Model file for the job. Use its own axes, mm. Face numbers are marked on the shaded views. A direction names the side the tool comes from. Give positions to 0.01 mm unless a question says otherwise; leave off trailing zeros. Write each loop counter-clockwise with the first axis right and the second up, starting at its lowest first coordinate (ties: lowest second). Pieces come first, ordered by that corner, then holes. Notation, with made-up numbers: (32.5, 5) - (38.5, 5) arc R29 cw to (38.5, 41) - close; hole circle Ø1 at (40.25, 60). An arc over 180 degrees is marked (long way). Use CSV: the item, a comma, the result in double quotes.
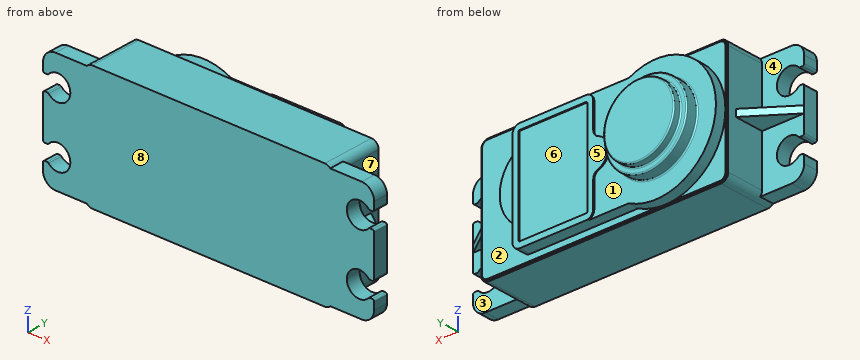
from build123d import *

# Parameters (mm, degrees)
CROQUIS1_W              = 41.6
CROQUIS1_H              = 20.6
SALIENTE_EXTRUIR1_DEPTH = 8.9
REDONDEO1_R             = 1.2
CROQUIS2_W              = 55.8
CROQUIS2_H              = 19.8
SALIENTE_EXTRUIR2_DEPTH = 2.45
REDONDEO2_R             = 2.1
CORTAR_EXTRUIR1_DEPTH   = 2.45
REDONDEO3_R             = 0.3
SALIENTE_EXTRUIR3_DEPTH = 0.2
CHAFL_N1_SIZE           = 0.1
SALIENTE_EXTRUIR4_DEPTH = 1.8
REDONDEO5_R             = 1.2
SALIENTE_EXTRUIR5_DEPTH = 0.2
CROQUIS11_R             = 6.95
SALIENTE_EXTRUIR6_DEPTH = 2
REDONDEO6_R             = 0.2
CROQUIS12_R             = 5.95
SALIENTE_EXTRUIR7_DEPTH = 1.3
REDONDEO7_R             = 0.2
SALIENTE_EXTRUIR8_DEPTH = 0.58


with BuildPart() as part:
    # Croquis1 → Saliente-Extruir1 (new body)
    with BuildSketch(Plane(origin=(0, 0, 0), x_dir=(1, 0, 0), z_dir=(0, 1, 0))):
        Rectangle(CROQUIS1_W, CROQUIS1_H)
    extrude(amount=SALIENTE_EXTRUIR1_DEPTH)

    # Redondeo1
    redondeo1_edges = [part.edges().sort_by_distance(p)[0] for p in [
        (20.8, 4.45, 10.3),
        (-20.8, 4.45, 10.3),
        (-20.8, 4.45, -10.3),
        (20.8, 4.45, -10.3),
    ]]
    fillet(redondeo1_edges, radius=REDONDEO1_R)

    # Croquis2 → Saliente-Extruir2 (add)
    with BuildSketch(Plane.XZ):
        Rectangle(CROQUIS2_W, CROQUIS2_H)
    extrude(amount=-SALIENTE_EXTRUIR2_DEPTH)

    # Redondeo2
    redondeo2_edges = [part.edges().sort_by_distance(p)[0] for p in [
        (-27.9, 1.225, -9.9),
        (-27.9, 1.225, 9.9),
        (27.9, 1.225, 9.9),
        (27.9, 1.225, -9.9),
    ]]
    fillet(redondeo2_edges, radius=REDONDEO2_R)

    # Croquis3 → Cortar-Extruir1 (cut)
    with BuildSketch(Plane.XZ):
        with BuildLine():
            Line((27.04924225, 6.3), (27.9, 6.3))
            Line((27.9, 6.3), (27.9, 3.7))
            Line((27.9, 3.7), (27.04924225, 3.7))
            ThreePointArc((27.04924225, 3.7), (23.3, 5), (27.04924225, 6.3))
        make_face()
        with BuildLine():
            Line((27.9, -6.3), (27.9, -3.7))
            Line((27.9, -3.7), (27.04924225, -3.7))
            ThreePointArc((27.04924225, -3.7), (23.3, -5), (27.04924225, -6.3))
            Line((27.04924225, -6.3), (27.9, -6.3))
        make_face()
        with BuildLine():
            Line((-27.04924225, -6.3), (-27.9, -6.3))
            Line((-27.9, -6.3), (-27.9, -3.7))
            Line((-27.9, -3.7), (-27.04924225, -3.7))
            ThreePointArc((-27.04924225, -3.7), (-23.3, -5), (-27.04924225, -6.3))
        make_face()
        with BuildLine():
            Line((-27.9, 6.3), (-27.9, 3.7))
            Line((-27.9, 3.7), (-27.04924225, 3.7))
            ThreePointArc((-27.04924225, 3.7), (-23.3, 5), (-27.04924225, 6.3))
            Line((-27.04924225, 6.3), (-27.9, 6.3))
        make_face()
    extrude(amount=-CORTAR_EXTRUIR1_DEPTH, mode=Mode.SUBTRACT)

    # Redondeo3
    redondeo3_edges = [part.edges().sort_by_distance(p)[0] for p in [
        (27.04924225, 1.225, 3.7),
        (27.04924225, 1.225, 6.3),
        (27.9, 1.225, 6.3),
        (27.9, 1.225, 3.7),
        (27.9, 1.225, -6.3),
        (27.04924225, 1.225, -6.3),
        (27.04924225, 1.225, -3.7),
        (27.9, 1.225, -3.7),
        (-27.9, 1.225, 6.3),
        (-27.04924225, 1.225, 6.3),
        (-27.04924225, 1.225, 3.7),
        (-27.9, 1.225, 3.7),
        (-27.9, 1.225, -6.3),
        (-27.9, 1.225, -3.7),
        (-27.04924225, 1.225, -3.7),
        (-27.04924225, 1.225, -6.3),
    ]]
    fillet(redondeo3_edges, radius=REDONDEO3_R)

    # Croquis4 → Saliente-Extruir3 (add)
    with BuildSketch(Plane(origin=(0, 8.9, 0), x_dir=(1, 0, 0), z_dir=(0, 1, 0))):
        with BuildLine():
            Line((20.6, -9.1), (20.6, 9.1))
            ThreePointArc((20.6, 9.1), (20.307106781, 9.807106781), (19.6, 10.1))
            Line((19.6, 10.1), (-19.6, 10.1))
            ThreePointArc((-19.6, 10.1), (-20.307106781, 9.807106781), (-20.6, 9.1))
            Line((-20.6, 9.1), (-20.6, -9.1))
            ThreePointArc((-20.6, -9.1), (-20.307106781, -9.807106781), (-19.6, -10.1))
            Line((-19.6, -10.1), (19.6, -10.1))
            ThreePointArc((19.6, -10.1), (20.307106781, -9.807106781), (20.6, -9.1))
        make_face()
    extrude(amount=SALIENTE_EXTRUIR3_DEPTH)

    # Chaflán1
    chafl_n1_edges = [part.edges().sort_by_distance(p)[0] for p in [
        (20.307106781, 9.1, -9.807106781),
        (0, 9.1, -10.1),
        (-20.307106781, 9.1, -9.807106781),
        (-20.6, 9.1, 0),
        (-20.307106781, 9.1, 9.807106781),
        (0, 9.1, 10.1),
        (20.307106781, 9.1, 9.807106781),
        (20.6, 9.1, 0),
    ]]
    chamfer(chafl_n1_edges, length=CHAFL_N1_SIZE)

    # Croquis6 → Saliente-Extruir4 (add)
    with BuildSketch(Plane(origin=(0, 9.1, 0), x_dir=(1, 0, 0), z_dir=(0, 1, 0))):
        with BuildLine():
            Line((13.6, 5), (13.6, 9))
            Line((13.6, 9), (-5.816333345, 9))
            ThreePointArc((-5.816333345, 9), (-20.5, 0), (-5.816333345, -9))
            Line((-5.816333345, -9), (13.6, -9))
            Line((13.6, -9), (13.6, -5))
            ThreePointArc((13.6, -5), (15.94, 0), (13.6, 5))
        make_face()
    extrude(amount=SALIENTE_EXTRUIR4_DEPTH)

    # Redondeo5
    redondeo5_edges = [part.edges().sort_by_distance(p)[0] for p in [
        (13.6, 10, -9),
        (13.6, 10, 9),
    ]]
    fillet(redondeo5_edges, radius=REDONDEO5_R)

    # Croquis10 → Saliente-Extruir5 (add)
    with BuildSketch(Plane(origin=(0, 10.9, 0), x_dir=(1, 0, 0), z_dir=(0, 1, 0))):
        with BuildLine():
            Line((13.6, 7.8), (13.6, -7.8))
            ThreePointArc((13.6, -7.8), (13.248528137, -8.648528137), (12.4, -9))
            Line((12.4, -9), (1.2, -9))
            ThreePointArc((1.2, -9), (0.351471863, -8.648528137), (0, -7.8))
            Line((0, -7.8), (0, -3.5))
            ThreePointArc((0, -3.5), (-0.223519835, -2.802514168), (-0.810810811, -2.364864865))
            ThreePointArc((-0.810810811, -2.364864865), (-2.5, 0), (-0.810810811, 2.364864865))
            ThreePointArc((-0.810810811, 2.364864865), (-0.223519835, 2.802514168), (0, 3.5))
            Line((0, 3.5), (0, 7.8))
            ThreePointArc((0, 7.8), (0.351471863, 8.648528137), (1.2, 9))
            Line((1.2, 9), (12.4, 9))
            ThreePointArc((12.4, 9), (13.248528137, 8.648528137), (13.6, 7.8))
        make_face()
        with BuildLine():
            Line((12.4, 8), (1.2, 8))
            ThreePointArc((1.2, 8), (1.058578644, 7.941421356), (1, 7.8))
            Line((1, 7.8), (1, -7.8))
            ThreePointArc((1, -7.8), (1.058578644, -7.941421356), (1.2, -8))
            Line((1.2, -8), (12.4, -8))
            ThreePointArc((12.4, -8), (12.541421356, -7.941421356), (12.6, -7.8))
            Line((12.6, -7.8), (12.6, 7.8))
            ThreePointArc((12.6, 7.8), (12.541421356, 7.941421356), (12.4, 8))
        make_face(mode=Mode.SUBTRACT)
    extrude(amount=SALIENTE_EXTRUIR5_DEPTH)

    # Croquis11 → Saliente-Extruir6 (add)
    with BuildSketch(Plane(origin=(0, 10.9, 0), x_dir=(1, 0, 0), z_dir=(0, 1, 0))):
        with Locations((-10.4, 0)):
            Circle(CROQUIS11_R)
    extrude(amount=SALIENTE_EXTRUIR6_DEPTH)

    # Redondeo6
    redondeo6_edges = [part.edges().sort_by_distance(p)[0] for p in [
        (-17.35, 10.9, 0),
        (-17.35, 12.9, 0),
    ]]
    fillet(redondeo6_edges, radius=REDONDEO6_R)

    # Croquis12 → Saliente-Extruir7 (add)
    with BuildSketch(Plane(origin=(0, 12.9, 0), x_dir=(1, 0, 0), z_dir=(0, 1, 0))):
        with Locations((-10.4, 0)):
            Circle(CROQUIS12_R)
    extrude(amount=SALIENTE_EXTRUIR7_DEPTH)

    # Redondeo7
    redondeo7_edges = [part.edges().sort_by_distance(p)[0] for p in [
        (-16.35, 12.9, 0),
        (-16.35, 14.2, 0),
    ]]
    fillet(redondeo7_edges, radius=REDONDEO7_R)

    # Croquis13 → Saliente-Extruir8 (add, symmetric)
    with BuildSketch(Plane.XY):
        Polygon((20.8, 2.45), (27.9, 2.45), (20.8, 7.45), align=None)
        Polygon((-27.9, 2.45), (-20.8, 2.45), (-20.8, 7.45), align=None)
    extrude(amount=SALIENTE_EXTRUIR8_DEPTH, both=True)


solid = part.part
(1) Pull direction X, two halves, no side cores. Call the marked faces 6, 7 and 8: released by +X, released by -X, zero draft, split by the parting line, or undercut.
Checked values:
face 6,"undercut"
face 7,"released by +X"
face 8,"zero draft"
(2) Flat gauge pins, fed straight in: P1, Ø6, axis at x = 22.5, z = 4, coming from the +Y side; P2, Ø1.5, axis at x = -23, y = 4.5, coming from the +Z side; P3, Ø2, axis at x = -23, y = 1, coming from the -Z side. Where does each tip first touch, or does it go through?
Checked values:
P1,"stops at y = 9.1"
P2,"stops at z = 0.58"
P3,"stops at z = -9.9"
(3) Saw through at B-B, the plane x = 24. List the corners of the cut face in (y, z), then the cut area to 3 significant figures.
Checked values:
outline,"(0, -9.9) - (2.45, -9.9) - (2.45, -6.57) - (0, -6.57) - close; (0, -3.43) - (2.45, -3.43) - (2.45, -0.58) - (5.2, -0.58) - (5.2, 0.58) - (2.45, 0.58) - (2.45, 3.43) - (0, 3.43) - close; (0, 6.57) - (2.45, 6.57) - (2.45, 9.9) - (0, 9.9) - close"
area,"36.4 mm^2"
(4) 3-axis set-ups, long thin cutter, end or side, ignore diameter. For the marked faces 1, 2, 3, 4 and 5: which of +Z, -Z, +X, -X, +Y, -Y reach the whole face in a straight line?
Checked values:
face 1,"+Y"
face 2,"+X, +Y"
face 3,"-Z, +X, +Y"
face 4,"+Z, -X, +Y"
face 5,"+Z, -Z, +X, +Y"
(5) Wall check: probe 1 along Z at (x, y) = (25.4, 1.95); probe 2 along X at (y, z) = (11, -2.25); probe 3 along Y at (x, z) = (-4.5, -8.5). Give the ranges that are in metal, low to high. Write a range as [from, to].
Checked values:
probe 1,"z = [-9.9, -7.1], [-2.9, 2.9], [7.1, 9.9]"
probe 2,"x = [-17, -3.8], [-1.09, 1], [12.6, 13.6]"
probe 3,"y = [0, 10.9]"
(6) Saw through at C-C, the plane y = 3.5. List the corners of the cut face in (x, z), then the cut area to 3 significant figures.
Checked values:
outline,"(-26.41, -0.58) - (-20.8, -0.58) - (-20.8, -9.1) arc R1.2 ccw to (-19.6, -10.3) - (19.6, -10.3) arc R1.2 ccw to (20.8, -9.1) - (20.8, -0.58) - (26.41, -0.58) - (26.41, 0.58) - (20.8, 0.58) - (20.8, 9.1) arc R1.2 ccw to (19.6, 10.3) - (-19.6, 10.3) arc R1.2 ccw to (-20.8, 9.1) - (-20.8, 0.58) - (-26.41, 0.58) - close"
area,"869 mm^2"
(7) Saw through at D-D, the plane x = 5. List the corners of the cut face in (y, z), then the cut area to 3 significant figures.
Checked values:
outline,"(0, -10.3) - (8.9, -10.3) - (8.9, -10.1) - (9, -10.1) - (9.1, -10) - (9.1, -9) - (11.1, -9) - (11.1, -8) - (10.9, -8) - (10.9, 8) - (11.1, 8) - (11.1, 9) - (9.1, 9) - (9.1, 10) - (9, 10.1) - (8.9, 10.1) - (8.9, 10.3) - (0, 10.3) - close"
area,"220 mm^2"
